Autodesk Fusion 360 part; units mm, degrees
sketch "Sketch1" plane through (0, 0, 0) normal (1, 0, 0) x (0, 1, 0)
  circle A0 centre (0, 0) radius 100
  dimension "d1" = 200
extrude "Extrude1" add sketch "Sketch1" along normal blind 4
sketch "Sketch2" plane through (4, 0, 0) normal (1, 0, 0) x (0, 1, 0)
  circle A0 centre (0, 0) radius 100
  circle A1 centre (0, 0) radius 26.5
  circle A2 centre (0, 0) radius 29.5
  dimension "d4" = 53
  dimension "d5" = 3
extrude "Extrude2" add sketch "Sketch2" along normal blind 27.5 contours A2
extrude "Extrude3" cut 1 faces at (4, -6.4753, 6.0082) along direction (-1, 0, 0) blind 40
mirror "Mirror1" about plane through (31.5, 0, 0) normal (1, 0, 0) of bodies 1 merged
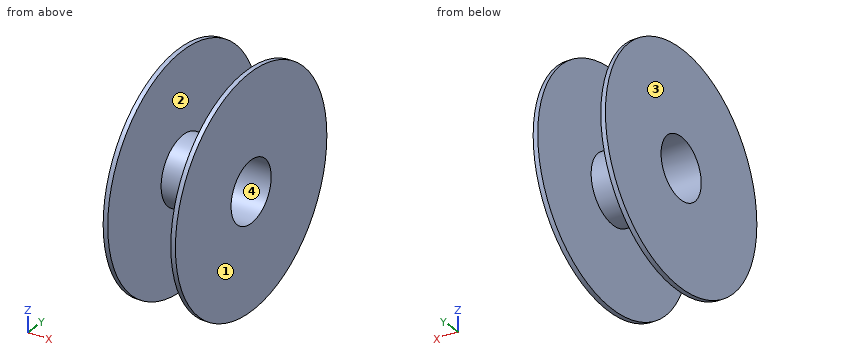
Model file for the job. Use its own axes, mm. Face numbers are marked on the shaded views. Give positions to 0.01 mm unless a question says otherwise; leave off trailing zeros. Order: outer loops, then holes, each group sorted by start corner. A loop starts at its lowest first (then second) coordinate and runs counter-clockwise, first axis right, second up.
1) Saw through at C-C, the plane y = 65. Write the cut outline in (x, z), then the cut area to 3 significant figures.
2) Saw through at A-A, the plane z = 0. Write the cut outline in (x, y).
3) Saw through at D-D, the plane x = 42. Write the cut outline in (y, z).
4) Wall check: probe 1 along X at (y, z) = (3, -70); probe 2 along Z at (x, y) = (42, 0); probe 3 along Z at (x, y) = (6.5, 15). Give the ranges that are in metal, low to high.
5) Mould opens along X. For the marked faces 1, 2, 3 and 4 say: +X half, -X half, draft (parallel to the pull), parting line (faces both ways), or undercut.
6) Pin check, flat tips, straight feed: pin 1 (3 mm diameter, centred on x = 12, z = -5, fed in from -Y); pin 2 (1 mm diameter, centred on x = 33.5, z = 0, fed in from -Y); pin 3 (12 mm diameter, centred on x = 34.5, z = 13.5, fed in from -Y). Stop position of each tip, or through.
Computed:
1. outline: (0, -75.99) - (4, -75.99) - (4, 75.99) - (0, 75.99) - close; (59, -75.99) - (63, -75.99) - (63, 75.99) - (59, 75.99) - close
1. area: 1,220 mm2
2. outline: (0, -100) - (4, -100) - (4, -29.5) - (59, -29.5) - (59, -100) - (63, -100) - (63, -26.5) - (0, -26.5) - close; (0, 26.5) - (63, 26.5) - (63, 100) - (59, 100) - (59, 29.5) - (4, 29.5) - (4, 100) - (0, 100) - close
3. outline: circle Ø59 at (0, 0); hole circle Ø53 at (0, 0)
4. probe 1: x = 0 to 4, 59 to 63
4. probe 2: z = -29.5 to -26.5, 26.5 to 29.5
4. probe 3: z = -25.4 to -21.85, 21.85 to 25.4
5. face 1: +X half
5. face 2: undercut
5. face 3: -X half
5. face 4: draft
6. pin 1: stops at y = -29.29
6. pin 2: stops at y = -29.5
6. pin 3: stops at y = -28.53
